Can you work these out from the model? Positions are in its coordinate system, mm. A direction names the side the tool comes from. Round coordinates to 2 decimals unless told otherwise and drop trailing zeros. Loops run counter-clockwise (first coordinate to the right, second up) from the corner with the lowest first, then second, coordinate; pieces in that order, holes last. Notation, with made-up numbers: M 47.5,18.25 L 68.5,18.25 A26 cw 68.5,39.25 Z; hole C -7.75,-31.75 d8. An arc over 180 degrees is marked long. Return JSON: item names as keys, results as strings.
Autodesk Fusion 360 part; units mm, degrees
sketch "Sketch1" plane through (0, 0, 0) normal (0, 0, 1) x (1, 0, 0)
  line L0 (0, 0) -> (0, 31.75)
  line L1 (0, 31.75) -> (10, 31.75)
  line L2 (10, 31.75) -> (10, 15.875)
  line L3 (10, 15.875) -> (12, 15.875)
  line L4 (0, 0) -> (-3, 0)
  line L5 (-3, 0) -> (-3, 35)
  line L6 (-3, 35) -> (13, 35)
  line L7 (13, 35) -> (13, 17.5)
  line L8 (13, 17.5) -> (10, 17.5)
  circle A0 centre (31.0292, 24.0805) radius 4.572
  circle A1 centre (31.0292, 24.0805) radius 6.572
  line L9 (13, 17.5) -> (31.0468, 17.5)
  line L10 (31.0468, 17.5) -> (31.0468, 19.5)
  line L11 (31.0468, 19.5) -> (13, 19.5)
  line L12 (13, 19.5) -> (13, 17.5)
  line L13 (31.0292, 28.6525) -> (12.2404, 28.6525)
  line L14 (12.2404, 28.6525) -> (12.2404, 30.6525)
  line L15 (12.2404, 30.6525) -> (31.0292, 30.6525)
  line L16 (31.0292, 30.6525) -> (31.0292, 28.6525)
  line L17 (38, 25) -> (24.0584, 25)
  line L18 (24.0584, 25) -> (24.0584, 23.1611)
  line L19 (24.0584, 23.1611) -> (38, 23.1611)
  line L20 (38, 23.1611) -> (38, 25)
  line L21 (38, 25) -> (24.0584, 23.1611) construction
  line L22 (24.0584, 25) -> (38, 23.1611) construction
  point P0 (31.0292, 24.0805)
  dimension "d1" = 31.75
  dimension "d2" = 10
  dimension "d3" = 15.875
  dimension "d4" = 2
  dimension "d5" = 9.144
  dimension "d6" = 2
  dimension "d11" = 2
  dimension "d12" = 2
extrude "Extrude3" add sketch "Sketch1" along normal blind 15 contours L0 L1 L2 L4 L5 L6 L7 L8 L12 L13 L14 L15 | L7 A1 L9 L10 L11 L12 | L7 A1 L13 L15 | L7 L13 L14 L15 | A1 L13 L16 | A0 A1 L16 L17 | A1 L10 L11 | A0 A1 L10 L11 L19 | A0 A1 L13 L17 | A0 A1 L17 L19 picked at (25.8467, 24.7963)
sketch "Sketch3" plane through (0, 0, 10) normal (0, 0, 1) x (-1, 0, 0)
  line L0 (-13, -17.5) -> (-13, -35)
  line L1 (-13, -35) -> (3, -35)
  line L2 (3, -35) -> (3, 0)
  line L3 (3, 0) -> (0, 0)
  line L4 (0, 0) -> (0, -31.75)
  line L5 (0, -31.75) -> (-10, -31.75)
  line L6 (-10, -31.75) -> (-10, -17.5)
  line L7 (-10, -17.5) -> (-13, -17.5)
  circle A0 centre (-17.7478, -24.1114) radius 4.572
sketch "Sketch4" plane through (0, 0, 10) normal (0, 0, 1) x (-1, 0, 0)
  line L0 (-13, -17.5) -> (-13, -35)
  line L1 (-13, -35) -> (3, -35)
  line L2 (3, -35) -> (3, 0)
  line L3 (3, 0) -> (0, 0)
  line L4 (0, 0) -> (0, -31.75)
  line L5 (0, -31.75) -> (-10, -31.75)
  line L6 (-10, -31.75) -> (-10, -17.5)
  line L7 (-10, -17.5) -> (-13, -17.5)
  circle A0 centre (-17.7478, -24.1114) radius 4.572
  circle A1 centre (-17.7478, -24.1114) radius 6.572
  line L8 (-17.5, -22.5) -> (-17.5, -16.7493)
fillet "Fillet1" radius 4.5 2 edges at (13, 19.5, 7.5) (13, 28.6525, 7.5)
fillet "Fillet2" radius 3 2 edges at (13, 35, 7.5) (-3, 35, 7.5)
Q1. If I drill on line 1 along X through (y, z) = (20, 13); line 2 along X through (y, z) = (20.5, 2.75); line 3 along X through (y, z) = (29, 13.5), over which ranges is the centre line in solid material (lowest first)?
Results:
{"line 1": "x = -3 to 0, 10 to 15.44, 25.88 to 28.97, 33.09 to 36.18", "line 2": "x = -3 to 0, 10 to 14.67, 25.52 to 28.19, 33.87 to 36.54", "line 3": "x = -3 to 0, 10 to 35.39"}
Q2. Suppose I cut it at D-D, the plane x = 29.5. Please give me the cut outline in (y, z).
Results:
{"outline": "M 17.5,0 L 19.77,0 L 19.77,15 L 17.5,15 Z; M 28.39,0 L 30.65,0 L 30.65,15 L 28.39,15 Z"}
Q3. Suppose I cut it at C-C, the plane y = 22. Please give me the cut outline in (x, z).
Results:
{"outline": "M -3,0 L 0,0 L 0,15 L -3,15 Z; M 10,0 L 13.47,0 L 13.47,15 L 10,15 Z; M 24.8,0 L 26.96,0 L 26.96,15 L 24.8,15 Z; M 35.1,0 L 37.26,0 L 37.26,15 L 35.1,15 Z"}
Q4. Suppose I cut it at A-A, the plane x = 24. Please give me the cut outline in (y, z), plus the area to 3 significant figures.
Results:
{"outline": "M 17.5,0 L 19.5,0 L 19.5,15 L 17.5,15 Z; M 28.65,0 L 30.65,0 L 30.65,15 L 28.65,15 Z", "area": "60.0 mm2"}
Q5. Thinking about a two-plate mould opening in X: for faces 6 (the cylindrical face through (35.395, 19.168, 7.395)), 7 (the flat face through (5, 31.75, 7)), 8 (the flat face through (12.7, 24.1, 15)), 9 (the flat face through (22, 28.652, 7)), which applies, pulls with the +X half, pulls with the -X half, needs draft (parallel to the pull), parting line crosses it, or undercut?
Results:
{"face 6": "pulls with the +X half", "face 7": "undercut", "face 8": "needs draft", "face 9": "undercut"}
Q6. I'm going to push flat-ended pins straight in: pin 1 Ø1.1 at (y, z) = (31.5, 7) entering from +X; pin 2 Ø6 at (y, z) = (17, 3.5) entering from +X; pin 3 Ø8 at (x, z) = (5, 7.5) entering from -Y; pin 4 Ø8 at (x, y) = (31.03, 24.08) entering from +Z. Where does each tip first touch, or does it pass through?
Results:
{"pin 1": "stops at x = 13", "pin 2": "stops at x = 36.18", "pin 3": "stops at y = 31.75", "pin 4": "passes through"}
Q7. On a 3-axis mill with a long thin cutter (end or side, diameter ignored), from which of +Z, -Z, +X, -X, +Y, -Y can I reach the whole of each face in a straight line? I mean faces 1 (the flat face through (21, 17.5, 7)), 2 (the flat face through (10, 25, 7)), 3 (the cylindrical face through (14.283, 20.853, 7.605)), 4 (the flat face through (22, 30.652, 7)), 5 (the flat face through (37, 25, 7)). Say none if no direction works.
Results:
{"face 1": "+Z, -Z, +X, -Y", "face 2": "+Z, -Z, -Y", "face 3": "+Z, -Z", "face 4": "+Z, -Z, +X, +Y", "face 5": "+Z, -Z, +X"}
